For this review, take the finished solid that the model builds, in its own axes (mm). A direction names the side the tool comes from. Round coordinates to 2 decimals unless told otherwise and drop trailing zeros. Order: outer loops, then holes, each group sorted by start corner. A loop starts at its lowest first (then second) coordinate and runs counter-clockwise, first axis right, second up. Notation, with made-up numbers: M -36.75,-21 L -27.75,-21 A26 ccw -27.75,8 Z; hole C 89.5,19.25 d4. An arc over 180 degrees is marked long. Use a Markdown table: item, result.
from build123d import *

# Parameters (mm, degrees)
F0_R     = 4
F1_DEPTH = 10
F2_W     = 15
F2_H     = 2
F3_DEPTH = 5
F4_R     = 2


with BuildPart() as f1:
    # F0 (on Top) → F1 (new body)
    with BuildSketch(Plane.XY):
        Circle(F0_R)
    extrude(amount=F1_DEPTH)

    # F2 (on face) → F3 (join)
    with BuildSketch(Plane.XY.offset(10)):
        with Locations((7.5, 0)):
            Rectangle(F2_W, F2_H)
    extrude(amount=-F3_DEPTH)

    # F4
    f4_edges = [f1.edges().sort_by_distance(p)[0] for p in [
        (15, 0, 10),
        (15, 0, 5),
    ]]
    fillet(f4_edges, radius=F4_R)


solid = f1.part
Q1. Machinability: for faces 1 (the flat face through (9, 1, 8)), 2 (the cylindrical face through (14.4, 0.01, 9.43)), 3 (the flat face through (9, -1, 8)), which of the approach directions +Z, -Z, +X, -X, +Y, -Y give a long, thin tool a straight path to every point of the face, cutting with its end or side? Answer none if there is none.
Determined:
| item | result |
|---|---|
| face 1 | +Z, -Z, +X, +Y |
| face 2 | +Z, +X, +Y, -Y |
| face 3 | +Z, -Z, +X, -Y |
Q2. Wall thickness on line 1 along Y through (x, z) = (12.25, 7.5); line 2 along Z through (x, y) = (8.25, 0.75); line 3 along X through (y, z) = (-1.5, 5): over which ranges is each line inside the solid? List them lowest first. Write a range as [from, to].
Determined:
| item | result |
|---|---|
| line 1 | y = [-1, 1] |
| line 2 | z = [5, 10] |
| line 3 | x = [-3.71, 3.71] |
Q3. Clearance check with flat-ended pins moving along their axes: pin 1 (1.5 mm diameter, centred on y = 1, z = 4.5, fed in from +X); pin 2 (4 mm diameter, centred on y = -2.5, z = 3.5, fed in from -X); pin 3 (1.5 mm diameter, centred on x = 11, z = 6.5, fed in from +Y). State where each tip first meets the part, or that it passes through.
Determined:
| item | result |
|---|---|
| pin 1 | stops at x = 13.97 |
| pin 2 | stops at x = -3.97 |
| pin 3 | stops at y = 1 |
Q4. Add section B-B (x = 5.25). Write out the cut boundary in (y, z).
Determined:
| item | result |
|---|---|
| outline | M -1,5 L 1,5 L 1,10 L -1,10 Z |
Q5. Add section D-D (x = 13.75). Write out the cut boundary in (y, z).
Determined:
| item | result |
|---|---|
| outline | M -1,5.15 L 1,5.15 L 1,9.85 L -1,9.85 Z |
Q6. Add section C-C (z = 3). Write out the cut boundary in (x, y).
Determined:
| item | result |
|---|---|
| outline | C 0,0 d8 |
Q7. Add section A-A (y = 0). Write out the cut boundary in (x, z).
Determined:
| item | result |
|---|---|
| outline | M -4,0 L 4,0 L 4,5 L 13,5 A2 ccw 15,7 L 15,8 A2 ccw 13,10 L -4,10 Z |
